Could you check a few things on this model? Use its own coordinates, in mm. Face numbers are marked on the shaded views. A direction names the side the tool comes from. Round coordinates to 2 decimals unless told otherwise and drop trailing zeros. Loops run counter-clockwise (first coordinate to the right, second up) from the corner with the lowest first, then second, coordinate; pieces in that order, holes last. Notation, with made-up numbers: M -9.5,19.25 L -0.5,19.25 A10 ccw -0.5,24.25 Z; hole C 5.25,5.25 d6. An arc over 180 degrees is marked long. Answer in a Markdown table with one row per item.
Autodesk Fusion 360 part; units mm, degrees
sketch "Sketch1" plane through (0, 0, 0) normal (0, 0, 1) x (1, 0, 0)
  line L0 (-29, 0) -> (29, 0)
  line L1 (29, 0) -> (29, -17)
  line L2 (29, -17) -> (-29, -17)
  line L3 (-29, -17) -> (-29, 0)
  line L4 (-31, 2) -> (31, 2)
  line L5 (31, 2) -> (31, 0)
  line L6 (31, 0) -> (-31, 0)
  line L7 (-31, 0) -> (-31, 2)
  line L8 (-27.55, -17) -> (27.55, -17)
  line L9 (27.55, -17) -> (27.55, -26)
  line L10 (27.55, -26) -> (-27.55, -26)
  line L11 (-27.55, -26) -> (-27.55, -17)
  line L12 (-20, -26) -> (20, -26)
  line L13 (20, -26) -> (20, -41)
  line L14 (20, -41) -> (-20, -41)
  line L15 (-20, -41) -> (-20, -26)
  line L16 (-42.5, 22) -> (42.5, 22)
  line L17 (42.5, 22) -> (42.5, 2)
  line L18 (42.5, 2) -> (-42.5, 2)
  line L19 (-42.5, 2) -> (-42.5, 22)
  line L20 (-42.5, -41) -> (-20, -41)
  line L21 (42.5, 2) -> (42.5, 22)
  line L22 (-39.5, 2) -> (-39.5, -41)
  line L23 (20, -41) -> (39.5, -41)
  line L24 (39.5, -41) -> (39.5, 2)
  line L25 (0, 2) -> (0, 22)
  line L26 (0, 2) -> (0, -41)
  dimension "d1" = 17
  dimension "d2" = 58
  dimension "d3" = 2
  dimension "d4" = 62
  dimension "d5" = 55.1
  dimension "d6" = 9
  dimension "d7" = 15
  dimension "d8" = 40
  dimension "d9" = 85
  dimension "d10" = 20
  dimension "d23" = 3
  dimension "d24" = 3
extrude "Extrude3" add sketch "Sketch1" along normal mid plane 65 contours L0 L4 L6 L7 L18 L26 | L0 L2 L3 L6 L8 L26 | L2 L3 L6 L7 L10 L11 L15 L18 L20 L22 | L0 L4 L5 L6 L18 L26 | L0 L1 L2 L6 L8 L26 | L1 L2 L5 L6 L9 L10 L13 L18 L23 L24 | L2 L8 L10 L11 L12 L26 | L2 L8 L9 L10 L12 L26 | L10 L12 L14 L15 L26 | L10 L12 L13 L14 L26
revolve "Revolve2" cut sketch "Sketch1" angle 360 about axis through (0, 2, 0) along (0, -1, 0) contours L0 L4 L6 L7 L18 L26 | L0 L2 L3 L6 L8 L26 | L2 L8 L10 L11 L12 L26 | L10 L12 L14 L15 L26
sketch "Sketch2" plane through (0, 2, 0) normal (0, 1, 0) x (-1, 0, 0)
  circle A0 centre (0, 0) radius 31
  line L0 (39.5, -32.5) -> (39.5, 32.5)
  line L1 (39.5, 32.5) -> (-39.5, 32.5)
  line L2 (-39.5, 32.5) -> (-39.5, -32.5)
  line L3 (-39.5, -32.5) -> (39.5, -32.5)
  line L4 (-39.5, 0.75) -> (-30.9909, 0.75)
  line L5 (-30.9909, 0.75) -> (-30.9909, -0.75)
  line L6 (-30.9909, -0.75) -> (-39.5, -0.75)
  line L7 (-39.5, -0.75) -> (-39.5, 0.75)
  line L8 (39.5, 0.75) -> (30.9909, 0.75)
  line L9 (30.9909, 0.75) -> (30.9909, -0.75)
  line L10 (30.9909, -0.75) -> (39.5, -0.75)
  line L11 (39.5, -0.75) -> (39.5, 0.75)
  line L12 (42.5, 0) -> (-42.5, 0)
  point P0 (28.9828, 11)
  dimension "d28" = 1.5
  dimension "d29" = 1.5
extrude "Extrude4" cut sketch "Sketch2" against normal blind 2 contours A0 L0 L10 L11 L12 | A0 L0 L8 L11 L12 | A0 L2 L4 L7 L12 | A0 L2 L6 L7 L12
sketch "Sketch3" plane through (0, 0, 0) normal (0, 1, 0) x (-1, 0, 0)
  circle A0 centre (0, 0) radius 29
  arc A1 (30.9909, 0.75) -> (-30.9909, 0.75) centre (0, 0) ccw
  line L0 (-30.9909, 0.75) -> (-39.5, 0.75)
  line L1 (-39.5, 0.75) -> (-39.5, -0.75)
  line L2 (-39.5, -0.75) -> (-30.9909, -0.75)
  arc A2 (-30.9909, -0.75) -> (30.9909, -0.75) centre (0, 0) ccw
  line L3 (30.9909, -0.75) -> (39.5, -0.75)
  line L4 (39.5, -0.75) -> (39.5, 0.75)
  line L5 (39.5, 0.75) -> (30.9909, 0.75)
  line L6 (28.9828, -11) -> (30.5941, -5)
  line L7 (30.5941, -5) -> (28.6521, -4.4785)
  line L8 (28.6521, -4.4785) -> (27.0407, -10.4785)
  line L9 (27.0407, -10.4785) -> (28.9828, -11)
  line L10 (-1.75, 0) -> (-22.5, 0)
  circle A3 centre (0, 0) radius 31
  line L11 (-30.5941, 5) -> (-28.6521, 4.4785)
  line L12 (-28.9828, 11) -> (-30.5941, 5)
  line L13 (-28.6521, 4.4785) -> (-27.0407, 10.4785)
  line L14 (-27.0407, 10.4785) -> (-28.9828, 11)
  line L15 (31, 0) -> (30.5941, -5)
  line L16 (0, 0) -> (31, 0)
  dimension "d35" = 6
  dimension "d37" = 360
  dimension "d41" = 5
extrude "Extrude5" cut sketch "Sketch3" against normal blind 13 contours A0 L11 L12 L14 | A0 L6 L7 L9
ref_plane "WorkPlane3" through (0, -9, 0) normal (0, 1, 0) x (0, 0, 1)
sketch "Sketch4" plane through (0, -9, 0) normal (0, 1, 0) x (1, 0, 0)
extrude "Extrude6" add 1 faces at (-13.1667, -26.6667, 32.5) along direction (0, 0, 1) blind 20
sketch "Sketch6" plane through (0, 0, 52.5) normal (0, 0, 1) x (-1, 0, 0)
  line L0 (39.5, 41) -> (-39.5, 41)
  line L1 (-39.5, 41) -> (-39.5, -2)
  line L2 (-39.5, -2) -> (39.5, -2)
  line L3 (39.5, -2) -> (39.5, 41)
  line L4 (-29.05, 41) -> (29.05, 41)
  line L5 (29.05, 41) -> (29.05, -2)
  line L6 (29.05, -2) -> (-29.05, -2)
  line L7 (-29.05, -2) -> (-29.05, 41)
  line L8 (29.05, 30) -> (39.5, 30)
  line L9 (-39.5, 30.6348) -> (-29.05, 30.6348)
  dimension "d44" = 58.1
extrude "Extrude7" add sketch "Sketch6" along normal blind 58.1 contours L0 L2 L4 L5 L6 L7
sketch "Sketch7" plane through (0, 2, 0) normal (0, 1, 0) x (-1, 0, 0)
  line L0 (-39.5, 0.75) -> (-30.9909, 0.75)
  arc A0 (30.9909, 0.75) -> (-30.9909, 0.75) centre (0, 0) ccw
  line L1 (30.9909, 0.75) -> (39.5, 0.75)
  line L2 (39.5, 0.75) -> (39.5, 52.5)
  line L3 (39.5, 52.5) -> (29.05, 52.5)
  line L4 (29.05, 52.5) -> (29.05, 110.6)
  line L5 (29.05, 110.6) -> (-29.05, 110.6)
  line L6 (-29.05, 110.6) -> (-29.05, 52.5)
  line L7 (-29.05, 52.5) -> (-39.5, 52.5)
  line L8 (-39.5, 52.5) -> (-39.5, 0.75)
  line L9 (-29.05, 52.5) -> (29.05, 52.5)
  circle A1 centre (0, 81.55) radius 19.05
  line L10 (-7.5, 64.0385) -> (7.5, 64.0385)
  line L11 (7.5, 64.0385) -> (7.5, 52.5)
  line L12 (7.5, 52.5) -> (-7.5, 52.5)
  line L13 (-7.5, 52.5) -> (-7.5, 64.0385)
  line L14 (0, 110.6) -> (0, 100.6)
  line L15 (0, 62.5) -> (0, 52.5)
  line L16 (-7.5, 52.5) -> (7.5, 52.5)
  line L17 (7.5, 52.5) -> (7.5, 40.9615)
  line L18 (7.5, 40.9615) -> (-7.5, 40.9615)
  line L19 (-7.5, 40.9615) -> (-7.5, 52.5)
  point P0 (0, 52.5)
  point P1 (-6.1183, 63.5093)
  dimension "d47" = 38.1
  dimension "d58" = 15
extrude "Extrude8" cut sketch "Sketch7" against normal up to surface (43 mm away) contours A1 L10 | A1 L10
fillet "Fillet1" radius 5 1 edges at (29.05, -19.5, 52.5)
fillet "Fillet2" radius 5 1 edges at (-29.05, -19.5, 52.5)
fillet "Fillet3" radius 5 4 edges at (-29.05, -19.5, 110.6) (29.05, -19.5, 110.6) (39.5, -19.5, -32.5) (-39.5, -19.5, -32.5)
fillet "Fillet4" radius 3 2 edges at (39.5, -19.5, 52.5) (-39.5, -19.5, 52.5)
extrude "Extrude9" cut sketch "Sketch7" against normal up to surface (43 mm away) contours L9 A1 L12 L13 L15 L16 | L9 L12 L16 L17 L18 L19 | L9 A1 L11 L12 L15 L16
equation "d44 = 1.5 in + 2 cm"
equation "d45 = 1.5 in + 2 cm"
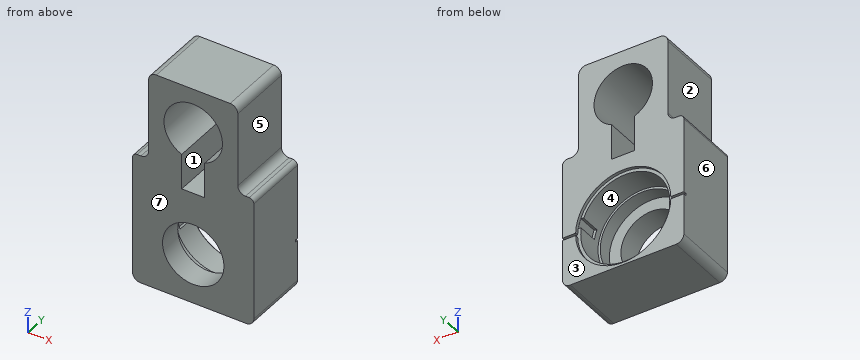
1) I want a section at D-D, the plane y = -18.5. Please give me the cut outline in (x, z).
Computed:
| item | result |
|---|---|
| outline | M -39.5,-27.5 A5 ccw -34.5,-32.5 L 34.5,-32.5 A5 ccw 39.5,-27.5 L 39.5,49.5 A3 ccw 36.5,52.5 L 34.05,52.5 A5 cw 29.05,57.5 L 29.05,105.6 A5 ccw 24.05,110.6 L -24.05,110.6 A5 ccw -29.05,105.6 L -29.05,57.5 A5 cw -34.05,52.5 L -36.5,52.5 A3 ccw -39.5,49.5 Z; hole C 0,0 d55.1; hole M -7.5,40.96 L 7.5,40.96 L 7.5,64.04 A19.05 ccw long -7.5,64.04 Z |
2) I need wall thicknesses on line 1 (Z direction, x = 1, y = -31); line 2 (Z direction, x = 0, y = -11.5); line 3 (X direction, y = -14.5, z = 60.5). Which ranges of each line are inside material? Lowest first, please.
Computed:
| item | result |
|---|---|
| line 1 | z = -32.5 to -19.97, 19.97 to 40.96, 100.57 to 110.6 |
| line 2 | z = -32.5 to -29, 29 to 40.96, 100.6 to 110.6 |
| line 3 | x = -29.05 to -7.5, 7.5 to 29.05 |
3) I want a section at B-B, the plane y = -29. Please give me the cut outline in (x, z), plus the area to 3 significant figures.
Computed:
| item | result |
|---|---|
| outline | M -39.5,-27.5 A5 ccw -34.5,-32.5 L 34.5,-32.5 A5 ccw 39.5,-27.5 L 39.5,49.5 A3 ccw 36.5,52.5 L 34.05,52.5 A5 cw 29.05,57.5 L 29.05,105.6 A5 ccw 24.05,110.6 L -24.05,110.6 A5 ccw -29.05,105.6 L -29.05,57.5 A5 cw -34.05,52.5 L -36.5,52.5 A3 ccw -39.5,49.5 Z; hole C 0,0 d40; hole M -7.5,40.96 L 7.5,40.96 L 7.5,64.04 A19.05 ccw long -7.5,64.04 Z |
| area | 7,350 mm² |
4) If we mould it in two halves opening along X, with no side actions, what happens to the marked faces 4, 5, 6 and 7? For each: released by +X, released by -X, zero draft, split by the parting line, or undercut.
Computed:
| item | result |
|---|---|
| face 4 | undercut |
| face 5 | released by +X |
| face 6 | released by -X |
| face 7 | zero draft |
5) I want a section at C-C, the plane x = 0. Please give me the cut outline in (y, z).
Computed:
| item | result |
|---|---|
| outline | M -41,-32.5 L 2,-32.5 L 2,-31 L 0,-31 L 0,-29 L -17,-29 L -17,-27.55 L -26,-27.55 L -26,-20 L -41,-20 Z; M -41,20 L -26,20 L -26,27.55 L -17,27.55 L -17,29 L 0,29 L 0,31 L 2,31 L 2,40.96 L -41,40.96 Z; M -41,100.6 L 2,100.6 L 2,110.6 L -41,110.6 Z |
6) Which directions (+Z, -Z, +X, -X, +Y, -Y) give clear straight access to the entire face, cutting with the end or side of a thin tool? Please do the marked faces 1, 2 and 3.
Computed:
| item | result |
|---|---|
| face 1 | +Y, -Y |
| face 2 | +Z, -X, +Y, -Y |
| face 3 | +Z, -Z, +X, -X, +Y |
7) I want a section at A-A, the plane z = 81.55. Please give me the cut outline in (x, y).
Computed:
| item | result |
|---|---|
| outline | M -29.05,-41 L -19.05,-41 L -19.05,2 L -29.05,2 Z; M 19.05,-41 L 29.05,-41 L 29.05,2 L 19.05,2 Z |
8) Will these pins go through, and if not, where does the flat tip stop? P1, Ø1.2, axis at x = 35.5, y = -23, coming from the +Z side; P2, Ø5, axis at y = -19.5, z = 85, coming from the +X side; P3, Ø1, axis at y = -34, z = 54.5, coming from the -X side.
Computed:
| item | result |
|---|---|
| P1 | stops at z = 52.5 |
| P2 | stops at x = 29.05 |
| P3 | stops at x = -30.48 |
